```python
from build123d import *

# Parameters (mm, degrees)
SKETCH_1_W          = 2.1
SKETCH_1_H          = 1
EXTRUDE_1_DEPTH     = 18
EXTRUDE_2_DEPTH     = 5
EXTRUDE_3_DEPTH     = 1
SKETCH_2_R          = 0.6
CUT_EXTRUDE_1_DEPTH = 20.270703153


with BuildPart() as part:
    # Sketch 1 → Extrude 1 (new body)
    with BuildSketch(Plane(origin=(0, 0, 0), x_dir=(0, 0, -1), z_dir=(1, 0, 0))):
        with BuildLine():
            Line((-3.5, 1), (-3.5, 0))
            Line((-3.5, 0), (-3.1, 0))
            ThreePointArc((-3.1, 0), (0, 3.1), (3.1, 0))
            Line((3.1, 0), (3.5, 0))
            Line((3.5, 0), (3.5, 1))
            Line((3.5, 1), (3.5, 4))
            Line((3.5, 4), (-3.5, 4))
            Line((-3.5, 4), (-3.5, 1))
        make_face()
        with Locations((-4.55, 0.5)):
            Rectangle(SKETCH_1_W, SKETCH_1_H)
        with Locations((4.55, 0.5)):
            Rectangle(SKETCH_1_W, SKETCH_1_H)
    extrude(amount=-EXTRUDE_1_DEPTH)

    # Sketch 1_6 → Extrude 2 (add)
    with BuildSketch(Plane(origin=(0, 0, 0), x_dir=(0, 0, -1), z_dir=(1, 0, 0))):
        with BuildLine():
            ThreePointArc((3.1, 0), (0, 3.1), (-3.1, 0))
            Line((-3.1, 0), (-1.5, 0))
            ThreePointArc((-1.5, 0), (0, 1.5), (1.5, 0))
            Line((1.5, 0), (3.1, 0))
        make_face()
    extrude(amount=-EXTRUDE_2_DEPTH)

    # Sketch 1_7 → Extrude 3 (add)
    with BuildSketch(Plane(origin=(0, 0, 0), x_dir=(0, 0, -1), z_dir=(1, 0, 0))):
        with BuildLine():
            ThreePointArc((1.5, 0), (0, 1.5), (-1.5, 0))
            Line((-1.5, 0), (1.5, 0))
        make_face()
    extrude(amount=-EXTRUDE_3_DEPTH)

    # Sketch 2 → Cut-Extrude 1 (cut, through all)
    with BuildSketch(Plane.XZ):
        with Locations(Location((-15, 4.329534947, 0), (0, 0, 270))):
            Circle(SKETCH_2_R)
        with Locations(Location((-4.5, 4.329534947, 0), (0, 0, 270))):
            Circle(SKETCH_2_R)
        with Locations(Location((-9, -4.420465053, 0), (0, 0, 270))):
            Circle(SKETCH_2_R)
    extrude(amount=-CUT_EXTRUDE_1_DEPTH, mode=Mode.SUBTRACT)


solid = part.part
```
Geometry: final body of the model. Coordinates: model frame, mm. A direction names the side the tool comes from. Coordinates: 2 decimals unless noted, no trailing zeros. Loops run counter-clockwise (first coordinate to the right, second up) from the corner with the lowest first, then second, coordinate; pieces in that order, holes last. Notation, with made-up numbers: (-7, 67) -> (29, 67) arc R14 cw to (29, 82) -> close; hole circle Ø10 at (6.25, 68). An arc over 180 degrees is marked (long way). Use a Markdown table: item, result. Add a question column.
(1) Pin query (flat end, axial travel): pin 1 Ø2.5 at (x, z) = (-11.5, 4.5) entering from +Y; pin 2 Ø1.6 at (x, z) = (-9, -4.42) entering from +Y; pin 3 Ø0.7 at (x, z) = (-4.5, 4.33) entering from +Y. Return the tip coordinate at first contact, or that it passes through.
(2) Section query B-B, the plane z = 0. Return loops of the section in (x, y), plus the area to 3 significant figures.
(3) Section query A-A, the plane x = -15. Return loops of the section in (y, z), plus the area to 3 significant figures.
(4) Mould query, pull axis Z, two halves, no side actions, for faces 1 (the cylindrical face through (-11.4, 3.1, 0.1)), 2 (the flat face through (-8.9, 0.5, -5.6)), 3 (the flat face through (-9, 4, 0)). Classes: pulls with the +Z half, pulls with the -Z half, needs draft (parallel to the pull), parting line crosses it, or undercut.
(5) Section query C-C, the plane z = 4. Return loops of the section in (x, y), plus the area to 3 significant figures.
(6) Access query for faces 4 (the flat face through (-5, 2, 0)), 5 (the flat face through (-9, 2, -3.5)), 6 (the flat face through (-9, 1, 5)), 7 (the flat face through (0, 2, 0)), 8 (the cylindrical face through (-14.82, 0.493, 3.757)). Directions: +Z, -Z, +X, -X, +Y, -Y. A direction counts if a zero-diameter tool reaches every point of the face in a straight line with its end or side. Return the directions, or none.
(7) Line query: line 1 along X through (y, z) = (0.9, -4.25); line 2 along Z through (x, y) = (-16, 3.3); line 3 along X through (y, z) = (0.4, -0.25). Output: solid intervals per line, ascending.
(8) Section query D-D, the plane x = -4.5. Return loops of the section in (y, z), plus the area to 3 significant figures.
Answer:
| question | item | result |
|---|---|---|
| 1 | pin 1 | stops at y = 4 |
| 1 | pin 2 | stops at y = 1 |
| 1 | pin 3 | passes through |
| 2 | outline | (-18, 3.1) -> (-5, 3.1) -> (-5, 1.5) -> (-1, 1.5) -> (-1, 0) -> (0, 0) -> (0, 4) -> (-18, 4) -> close |
| 2 | area | 25.7 mm^2 |
| 3 | outline | (0, -5.6) -> (1, -5.6) -> (1, -3.5) -> (4, -3.5) -> (4, 3.5) -> (1, 3.5) -> (1, 3.73) -> (0, 3.73) -> (0, 3.1) arc R3.1 cw to (0, -3.1) -> close; (0, 4.93) -> (1, 4.93) -> (1, 5.6) -> (0, 5.6) -> close |
| 3 | area | 15.9 mm^2 |
| 4 | face 1 | undercut |
| 4 | face 2 | pulls with the -Z half |
| 4 | face 3 | needs draft |
| 5 | outline | (-18, 0) -> (-15.5, 0) -> (-15.5, 1) -> (-18, 1) -> close; (-14.5, 0) -> (-5, 0) -> (-5, 1) -> (-14.5, 1) -> close; (-4, 0) -> (0, 0) -> (0, 1) -> (-4, 1) -> close |
| 5 | area | 16.0 mm^2 |
| 6 | face 4 | -X, -Y |
| 6 | face 5 | -Z, +X, -X, +Y |
| 6 | face 6 | +Z, +X, -X, +Y |
| 6 | face 7 | +Z, -Z, +X, +Y, -Y |
| 6 | face 8 | +Y, -Y |
| 7 | line 1 | x = -18 to -9.58, -8.42 to 0 |
| 7 | line 2 | z = -3.5 to 3.5 |
| 7 | line 3 | x = -1 to 0 |
| 8 | outline | (0, -5.6) -> (1, -5.6) -> (1, -3.5) -> (4, -3.5) -> (4, 3.5) -> (1, 3.5) -> (1, 3.73) -> (0, 3.73) -> (0, 1.5) arc R1.5 cw to (0, -1.5) -> close; (0, 4.93) -> (1, 4.93) -> (1, 5.6) -> (0, 5.6) -> close |
| 8 | area | 27.5 mm^2 |
